from build123d import *

# Parameters (mm, degrees)
EXTRUDE_1_DEPTH      = 0.5
EXTRUDE_1_DEPTH_BACK = 33.5
SKETCH_1_R           = 4.75
SKETCH_2_R           = 1.5
CUT_EXTRUDE_1_DEPTH  = 10
CUT_EXTRUDE_START    = -8
CUT_EXTRUDE_2_DEPTH  = 8


with BuildPart() as part:
    # 草图1 → 凸台-拉伸1 (new, two sides: drawn at the far end of the back side and taken through both)
    with BuildSketch(Plane.XY.offset(-EXTRUDE_1_DEPTH_BACK)):
        Circle(SKETCH_1_R)
    extrude(amount=EXTRUDE_1_DEPTH + EXTRUDE_1_DEPTH_BACK)

    # 草图2 → 切除-拉伸1 (cut)
    with BuildSketch(Plane(origin=(0, 0, -33.5), x_dir=(-1, 0, 0), z_dir=(0, 0, -1))):
        Circle(SKETCH_2_R)
    extrude(amount=-CUT_EXTRUDE_1_DEPTH, mode=Mode.SUBTRACT)

    # 草图3 → 切除-拉伸2 (cut)
    with BuildSketch(Plane.XY.offset(0.5).offset(CUT_EXTRUDE_START)):
        with BuildLine():
            Line((0.8, 1.268857754), (0.8, -1.268857754))
            ThreePointArc((0.8, -1.268857754), (-1.5, 0), (0.8, 1.268857754))
        make_face()
    extrude(amount=CUT_EXTRUDE_2_DEPTH, mode=Mode.SUBTRACT)


solid = part.part
Design review of the part built by this model. Coordinates are the model's own, in mm. A direction names the side the tool comes from. Coordinates: 2 decimals unless noted, no trailing zeros. Write each loop counter-clockwise with the first axis right and the second up, starting at its lowest first coordinate (ties: lowest second). Pieces come first, ordered by that corner, then holes. Notation, with made-up numbers: (52.25, 39.25) -> (83.25, 39.25) arc R24 cw to (83.25, 62.25) -> close; hole circle Ø10 at (13, 12). An arc over 180 degrees is marked (long way). Write each question's results on one line, items separated by ' | '. Start each with the question number.
(1) Take a section at B-B on y = 0. Write out the cut boundary in (x, z).
(2) The part is to be moulded in two halves that separate along Y. For faces 4 (the face through (-1.5, 0, -3.6)), 5 (the face through (2.192, -4.214, -16.738)), 6 (the face through (0, 0, -7.5)), 7 (the face through (1, 0, 0.5)), say which applies: pulls with the +Y half, pulls with the -Y half, needs draft (parallel to the pull), parting line crosses it, or undercut.
(3) Take a section at D-D on z = -8. Write out the cut boundary in (x, y).
(4) Tool access review of faces 1 (the face through (0, 0, -23.5)), 2 (the face through (2, 0, -33.5)), 3 (the face through (0.8, 0, -4)): name each direction out of +Z, -Z, +X, -X, +Y, -Y from which nothing blocks a thin tool from reaching the whole face with its end or side.
(5) Take a section at A-A on x = 0. Write out the cut boundary in (y, z), and give its area (3 significant figures).
(6) Clearance check with flat-ended pins moving along their axes: P1, Ø1.5, axis at x = 0.5, y = -0.5, coming from the -Z side; P2, Ø1, axis at x = -0.5, y = 0, coming from the +Z side; P3, Ø1, axis at y = -3, z = -23.5, coming from the +X side. State where each tip first meets the part, or that it passes through.
(7) For line 1 along Y through (x, z) = (0, -28.75); line 2 along Z through (x, y) = (1.25, 0.75); line 3 along Y through (x, z) = (-0.75, -5), list the stretches that pass through material, from the lowest coordinate up. Write a range as from..to.
(8) Take a section at C-C on z = -2. Write out the cut boundary in (x, y), and give its area (3 significant figures).
Results found:
1) outline: (-4.75, -33.5) -> (-1.5, -33.5) -> (-1.5, -23.5) -> (1.5, -23.5) -> (1.5, -33.5) -> (4.75, -33.5) -> (4.75, 0.5) -> (0.8, 0.5) -> (0.8, -7.5) -> (-1.5, -7.5) -> (-1.5, 0.5) -> (-4.75, 0.5) -> close
2) face 4: undercut | face 5: parting line crosses it | face 6: undercut | face 7: needs draft
3) outline: circle Ø9.5 at (0, 0)
4) face 1: -Z | face 2: -Z, +X, -X, +Y, -Y | face 3: +Z
5) outline: (-4.75, -33.5) -> (-1.5, -33.5) -> (-1.5, -23.5) -> (1.5, -23.5) -> (1.5, -33.5) -> (4.75, -33.5) -> (4.75, 0.5) -> (1.5, 0.5) -> (1.5, -7.5) -> (-1.5, -7.5) -> (-1.5, 0.5) -> (-4.75, 0.5) -> close | area: 269 mm2
6) P1: stops at z = -23.5 | P2: stops at z = -7.5 | P3: stops at x = 4.04
7) line 1: y = -4.75..-1.5, 1.5..4.75 | line 2: z = -23.5..0.5 | line 3: y = -4.69..-1.3, 1.3..4.69
8) outline: circle Ø9.5 at (0, 0); hole (0.8, -1.27) -> (0.8, 1.27) arc R1.5 ccw (long way) to start | area: 65.1 mm2
